Can you work these out from the model? Positions are in its coordinate system, mm. Round coordinates to 2 decimals unless told otherwise and drop trailing zeros. Write each loop counter-clockwise with the first axis right and the second up, starting at its lowest first coordinate (ties: lowest second). Pieces come first, ordered by that corner, then holes. Notation, with made-up numbers: (-33.5, 26) -> (-9.5, 26) arc R30 cw to (-9.5, 54) -> close; hole circle Ø4 at (23.5, 71.25). An arc over 180 degrees is marked (long way). Use CSV: the item, a comma, the result in double quotes.
Autodesk Inventor part; units mm, degrees
ref_plane "YZ Plane" through (0, 0, 0) normal (1, 0, 0) x (0, 1, 0)
ref_plane "XZ Plane" through (0, 0, 0) normal (0, 1, 0) x (-1, 0, 0)
ref_plane "XY Plane" through (0, 0, 0) normal (0, 0, 1) x (1, 0, 0)
sketch "Sketch1" plane through (0, 0, 0) normal (0, 0, 1) x (1, 0, 0)
  line L0 (-12.1708, 16.0073) -> (13.2292, 16.0073)
  line L1 (13.2292, 16.0073) -> (13.2292, -34.7927)
  line L2 (13.2292, -34.7927) -> (-12.1708, -34.7927)
  line L3 (-12.1708, -34.7927) -> (-12.1708, 16.0073)
  line L4 (11.9592, 14.7373) -> (-10.9008, 14.7373)
  line L5 (-10.9008, 14.7373) -> (-10.9008, -33.5227)
  line L6 (-10.9008, -33.5227) -> (11.9592, -33.5227)
  line L7 (11.9592, -33.5227) -> (11.9592, 14.7373)
  point P0 (0, 0)
  dimension "d0" = 25.4
  dimension "d1" = 50.8
  dimension "d2" = 1.27
extrude "Extrusion1" add sketch "Sketch1" along normal blind 457.2
sketch "Sketch2" plane through (-12.1708, 16.0073, 0) normal (0, 1, 0) x (1, 0, 0)
  circle A0 centre (12.7, -12.7) radius 1.7272
  line L0 (25.4, 0) -> (0, 0)
  line L1 (0, 0) -> (0, -457.2)
  point P0 (12.1708, 0)
  dimension "d5" = 3.4544
  dimension "d6" = 12.7
  dimension "d7" = 12.7
extrude "Extrusion2" cut sketch "Sketch2" against normal through all
pattern_linear "Rectangular Pattern1" count 46 spacing 25.4 along (0, 0, 1) of "Extrusion2"
equation "\"d3\" = d13"
equation "\"d10\" = d14"
equation "\"d13\" = 457.2"
equation "\"d14\" = d13"
properties part number "VersaFrame-18"
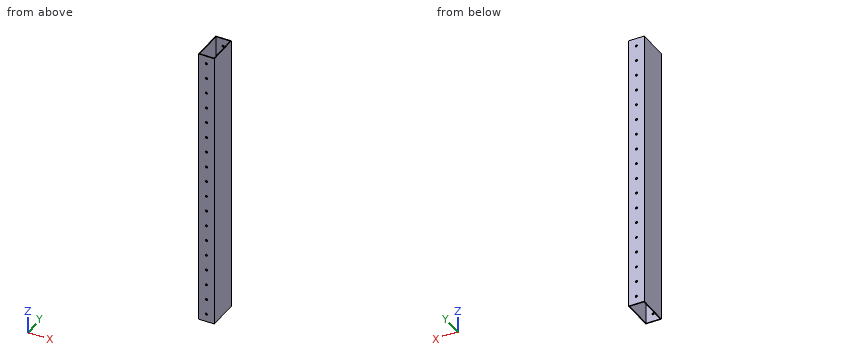
Q1. Will this pin go through, and if not, where does the flat tip stop? P1, Ø3, axis at x = 0.53, z = 38.1, coming from the +Y side.
Resolved:
P1,"passes through"
Q2. Please list where these lines run through material, in increasing order: probe 1 along Y at (x, z) = (2.25, 174.5); probe 2 along X at (y, z) = (-5.5, 352); probe 3 along X at (y, z) = (-34.4, 317.5).
Resolved:
probe 1,"y = -34.79 to -33.52, 14.74 to 16.01"
probe 2,"x = -12.17 to -10.9, 11.96 to 13.23"
probe 3,"x = -12.17 to -1.2, 2.26 to 13.23"
Q3. Suppose I cut it at B-B (z = 102.5). Write out the boundary of the cut face in (x, y).
Resolved:
outline,"(-12.17, -34.79) -> (13.23, -34.79) -> (13.23, 16.01) -> (-12.17, 16.01) -> close; hole (-10.9, -33.52) -> (11.96, -33.52) -> (11.96, 14.74) -> (-10.9, 14.74) -> close"
Q4. Suppose I cut it at A-A (y = 1). Write out the boundary of the cut face in (x, z).
Resolved:
outline,"(-12.17, 0) -> (-10.9, 0) -> (-10.9, 457.2) -> (-12.17, 457.2) -> close; (11.96, 0) -> (13.23, 0) -> (13.23, 457.2) -> (11.96, 457.2) -> close"
